from build123d import *

# Parameters (mm, degrees)
F0_R     = 13.9
F1_DEPTH = 217.8
F3_DEPTH = 35
F5_D     = 12.2
F7_DEPTH = 27.5


with BuildPart() as f1:
    # F0 (on Front) → F1 (new body, symmetric)
    with BuildSketch(Plane.XZ):
        Circle(F0_R)
    extrude(amount=F1_DEPTH, both=True)

    # F2 (on face) → F3 (cut)
    with BuildSketch(Plane.XZ.offset(217.8)):
        with BuildLine():
            ThreePointArc((13.9, 0), (13.8906348377, 0.5101605694), (13.8625519703, 1.0196336946))
            Line((13.8625519703, 1.0196336946), (13.8625519703, -1.0196336946))
            ThreePointArc((13.8625519703, -1.0196336946), (13.8906348377, -0.5101605694), (13.9, 0))
        make_face()
    extrude(amount=-F3_DEPTH, mode=Mode.SUBTRACT)

    # F5 (through all)
    with Locations(Plane.YZ.offset(13.8625519703)):
        with Locations((-204.8, 0)):
            Hole(F5_D / 2)

    # F6 (on face) → F7 (cut)
    with BuildSketch(Plane.XZ.offset(217.8)):
        with BuildLine():
            ThreePointArc((4.1, 13.2815661727), (0, 13.9), (-4.1, 13.2815661727))
            Line((-4.1, 13.2815661727), (-4.1, -13.2815661727))
            ThreePointArc((-4.1, -13.2815661727), (0, -13.9), (4.1, -13.2815661727))
            Line((4.1, -13.2815661727), (4.1, 13.2815661727))
        make_face()
    extrude(amount=-F7_DEPTH, mode=Mode.SUBTRACT)


solid = f1.part
Read the model definition and answer for the solid it produces. Units are mm, in the model's axes. A direction names the side the tool comes from. Coordinates: 2 decimals unless noted, no trailing zeros. Loops run counter-clockwise (first coordinate to the right, second up) from the corner with the lowest first, then second, coordinate; pieces in that order, holes last.
Q1. The part is cut by section C-C on y = 178.5. Write down the section's boundary in (x, z).
Q2. Which of the six approach directions +Z, -Z, +X, -X, +Y, -Y give full straight-line access (tool end or side, diameter ignored) to faces 1 (the face through (0, 217.8, 0)), 2 (the face through (4.1, -198, 0))?
Q3. The part is cut by section A-A on y = -204.8. Write down the section's boundary in (x, z), and give its area (3 significant figures).
Q4. The mould has two halves that part along Z. Classify faces 3 (the face through (12.84, -3.05, -5.32)), 4 (the face through (8.913, -198.706, 0.268)), 5 (the face through (-4.1, -198, 0)): +Z half, -Z half, draft (parallel to the pull), parting line (faces both ways), or undercut.
Q5. The part is cut by section B-B on x = 0. Write down the section's boundary in (y, z), and give its area (3 significant figures).
Q6. Each of these flat-tipped pins is pushed along its axis until it touches: pin 1 Ø10 at (y, z) = (-204.8, 0) entering from -X; pin 2 Ø4 at (x, z) = (-2, -5.5) entering from -Y; pin 3 Ø4 at (x, y) = (8.5, -67.5) entering from +Z; pin 4 Ø6 at (x, y) = (6.5, 169) entering from -Z. Where does it stop, or does it pass through?
Q7. Consider probe 1 along Y at (x, z) = (8, 0); probe 2 along Y at (x, z) = (-6.75, 1); probe 3 along Z at (x, y) = (8, -204.8). Determine where each line is inside the solid, lowest interval first.
Results below:
1. outline: circle Ø27.8 at (0, 0)
2. face 1: +Z, -Z, +X, -X, +Y
2. face 2: +Z, -Z, -Y
3. outline: (-12.49, -6.1) arc R13.9 ccw to (-4.1, -13.28) - (-4.1, -6.1) - close; (-12.49, 6.1) - (-4.1, 6.1) - (-4.1, 13.28) arc R13.9 ccw to start; (4.1, -13.28) arc R13.9 ccw to (12.49, -6.1) - (4.1, -6.1) - close; (4.1, 6.1) - (12.49, 6.1) arc R13.9 ccw to (4.1, 13.28) - close
3. area: 154 mm2
4. face 3: parting line
4. face 4: undercut
4. face 5: draft
5. outline: (-190.3, -13.9) - (217.8, -13.9) - (217.8, 13.9) - (-190.3, 13.9) - close
5. area: 11,300 mm2
6. pin 1: passes through
6. pin 2: stops at y = -190.3
6. pin 3: stops at z = 12.29
6. pin 4: stops at z = -13.45
7. probe 1: y = -217.8 to -210.9, -198.7 to 217.8
7. probe 2: y = -217.8 to -210.82, -198.78 to 217.8
7. probe 3: z = -11.37 to -6.1, 6.1 to 11.37
